Source: three-view drawing plus pictorial views. Frame: mm from the lowest corner of the part. A direction names the side the tool comes from. Round coordinates to 2 decimals unless told otherwise and drop trailing zeros. Loops run counter-clockwise (first coordinate to the right, second up) from the corner with the lowest first, then second, coordinate; pieces in that order, holes last. Notation, with made-up numbers: (27.25, 3.25) -> (38.25, 3.25) arc R34 ccw to (38.25, 37.25) -> close; hole circle Ø5 at (8.5, 54). An arc over 180 degrees is marked (long way). Answer as a JSON object with one key per item and string values. Group by question number.
Item 1: Section query C-C on z = 29. Return loops of the section in (x, y).
Item 2: Material intervals for line 1 (X direction, y = 35, z = 1.6); line 2 (Z direction, x = 15.5, y = 0.8); line 3 (X direction, y = 13.5, z = 8), sorted ascending. Write a range as [from, to].
Item 3: Draft query along X for the marked faces 4, 5 and 6. Return one class per face: released by +X, released by -X, zero draft, split by the parting line, or undercut.
Item 4: Section query B-B on x = 31. Return loops of the section in (y, z), and give its area (3 significant figures).
Item 5: Pin query (flat end, axial travel): pin 1 (3 mm diameter, centred on x = 46, z = 30, fed in from +Y); pin 2 (2 mm diameter, centred on y = 32.5, z = 9, fed in from -X); pin 3 (4.5 mm diameter, centred on x = 4.2, y = 20, fed in from +Z). Return the tip coordinate at first contact, or that it passes through.
Item 6: Set-up query: the marked faces 1, 2 and 3. Return all of +Z, -Z, +X, -X, +Y, -Y with unobstructed straight access to the full face (end or side cutting, diameter ignored); none if empty.
Item 7: Section query A-A on x = 15.5. Return loops of the section in (y, z), and give its area (3 significant figures).
Item 8: Section query D-D on y = 35. Return loops of the section in (x, z), and give its area (3 significant figures).
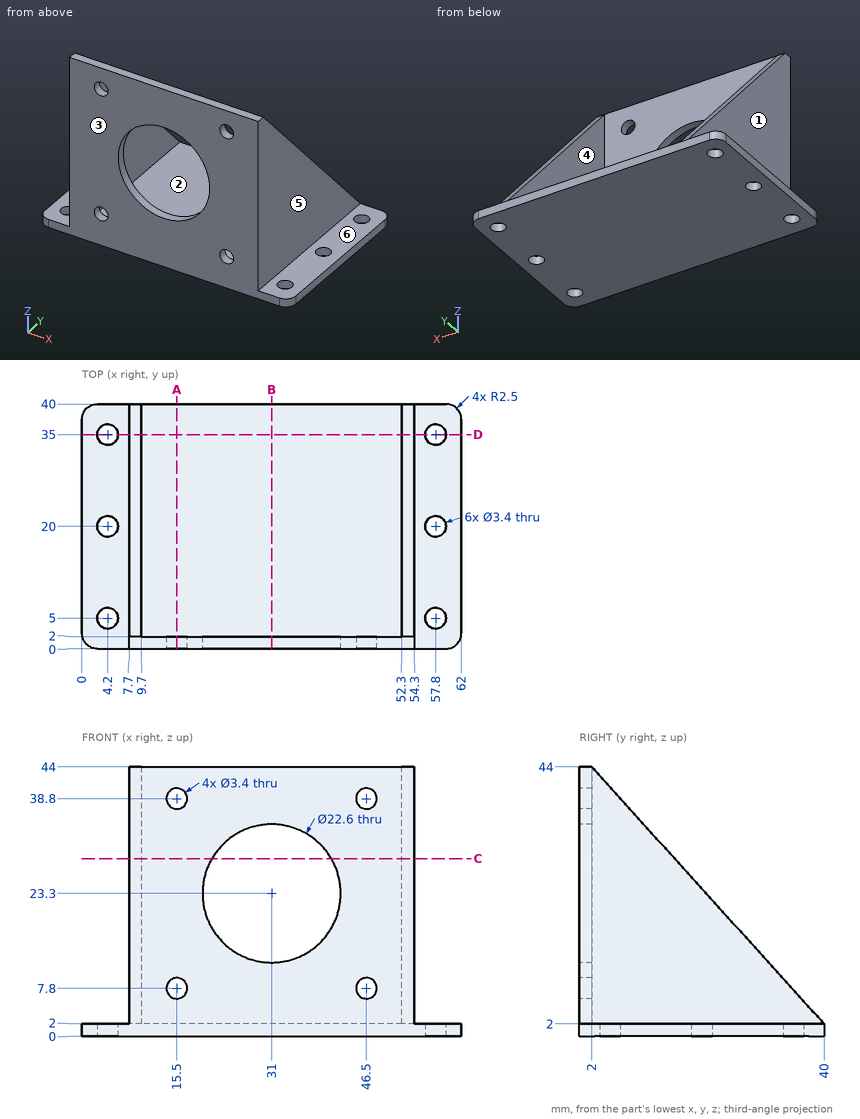
Solved:
{
 "1": {"outline": "(7.7, 0) -> (21.24, 0) -> (21.24, 2) -> (9.7, 2) -> (9.7, 15.57) -> (7.7, 15.57) -> close; (40.76, 0) -> (54.3, 0) -> (54.3, 15.57) -> (52.3, 15.57) -> (52.3, 2) -> (40.76, 2) -> close"},
 "2": {"line 1": "[0, 2.5], [5.9, 56.1], [59.5, 62]", "line 2": "[0, 6.1], [9.5, 37.1], [40.5, 44]", "line 3": "[7.7, 9.7], [52.3, 54.3]"},
 "3": {"face 4": "undercut", "face 5": "released by +X", "face 6": "zero draft"},
 "4": {"outline": "(0, 0) -> (40, 0) -> (40, 2) -> (2, 2) -> (2, 12) -> (0, 12) -> close; (0, 34.6) -> (2, 34.6) -> (2, 44) -> (0, 44) -> close", "area": "119 mm²"},
 "5": {"pin 1": "y = 2", "pin 2": "x = 7.7", "pin 3": "z = 2"},
 "6": {"face 1": "+Z, -X, +Y, -Y", "face 2": "+Z, +Y", "face 3": "+Z, -Z, +X, -X, -Y"},
 "7": {"outline": "(0, 0) -> (40, 0) -> (40, 2) -> (2, 2) -> (2, 6.1) -> (0, 6.1) -> close; (0, 9.5) -> (2, 9.5) -> (2, 37.1) -> (0, 37.1) -> close; (0, 40.5) -> (2, 40.5) -> (2, 44) -> (0, 44) -> close", "area": "150 mm²"},
 "8": {"outline": "(0, 0) -> (2.5, 0) -> (2.5, 2) -> (0, 2) -> close; (5.9, 0) -> (56.1, 0) -> (56.1, 2) -> (54.3, 2) -> (54.3, 7.53) -> (52.3, 7.53) -> (52.3, 2) -> (9.7, 2) -> (9.7, 7.53) -> (7.7, 7.53) -> (7.7, 2) -> (5.9, 2) -> close; (59.5, 0) -> (62, 0) -> (62, 2) -> (59.5, 2) -> close", "area": "133 mm²"}
}
